Could you check a few things on this model? Use its own coordinates, in mm. Face numbers are marked on the shaded views. A direction names the side the tool comes from. Round coordinates to 2 decimals unless told otherwise and drop trailing zeros. Order: outer loops, then holes, each group sorted by start corner. A loop starts at its lowest first (then second) coordinate and runs counter-clockwise, first axis right, second up.
```python
from build123d import *

# Parameters (mm, degrees)
SKETCH1_R           = 1.5
BOSS_EXTRUDE1_DEPTH = 2.5
BOSS_EXTRUDE2_DEPTH = 13
SKETCH3_R           = 1.6
CUT_EXTRUDE1_DEPTH  = 13


with BuildPart() as part:
    # Sketch1 → Boss-Extrude1 (new body)
    with BuildSketch(Plane(origin=(0, 0, 0), x_dir=(1, 0, 0), z_dir=(0, 1, 0))):
        Polygon((-58.606798355, 6.5), (-34.466582946, 0), (112.252986236, 0), (136.393201645, 6.5), (136.393201645, 13), (-58.606798355, 13), align=None)
        with Locations((-11.606798355, 9.25)):
            Circle(SKETCH1_R, mode=Mode.SUBTRACT)
        with Locations((89.393201645, 9.25)):
            Circle(SKETCH1_R, mode=Mode.SUBTRACT)
    extrude(amount=BOSS_EXTRUDE1_DEPTH)

    # Sketch2 → Boss-Extrude2 (add)
    with BuildSketch(Plane(origin=(0, 2.5, 0), x_dir=(1, 0, 0), z_dir=(0, 1, 0))):
        Polygon((-58.606798355, 6.5), (-34.466582946, 0), (10.033417054, 0), (10.033417054, 2.5), (-34.135896564, 2.5), (-57.956798355, 8.914021541), align=None)
        Polygon((136.393201645, 6.5), (112.252986236, 0), (67.752986236, 0), (67.752986236, 2.5), (111.922299855, 2.5), (135.743201645, 8.914021541), align=None)
    extrude(amount=BOSS_EXTRUDE2_DEPTH)

    # Sketch3 → Cut-Extrude1 (cut)
    with BuildSketch(Plane.XY):
        with Locations((-30.716582946, 9)):
            Circle(SKETCH3_R)
        with Locations((6.283417054, 9)):
            Circle(SKETCH3_R)
        with Locations((71.502986236, 9)):
            Circle(SKETCH3_R)
        with Locations((108.502986236, 9)):
            Circle(SKETCH3_R)
    extrude(amount=-CUT_EXTRUDE1_DEPTH, mode=Mode.SUBTRACT)


solid = part.part
```
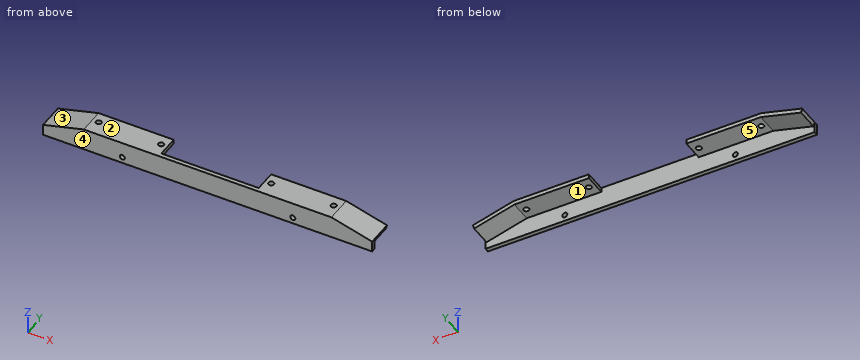
Q1. Imagine slicing it at A-A, the plane y = 9. Please give me the cut outline in (x, z), then the cut area to 3 significant figures.
Q2. I need wall thicknesses on L1, parallel to X at y = 1.3, z = -9.25; L2, parallel to Y at x = 98, z = -8.25; L3, parallel to Z at x = 74.5, y = 4.25. Which ranges of each line are inside material? Lowest first, please.
Q3. For the marked faces 1 and 2, which set-ups out of +Z, -Z, +X, -X, +Y, -Y let a thin tool reach every point of the face, with its end or its side?
Q4. Imagine slicing it at C-C, the plane x = 31.5. Please give me the cut outline in (y, z), then the cut area to 3 significant figures.
Q5. For P1, Ø4, axis at x = 19.5, z = -6, coming from the +Y side; P2, Ø1, axis at x = 106.5, y = 5, coming from the +Z side; P3, Ø6.5, axis at x = 100.5, y = 10, coming from the -Z side, each with a flat end and sliding along its axis, tell me the tip position at first contact or that it passes through.
Q6. Imagine slicing it at D-D, the plane x = -37. Please give me the cut outline in (y, z).
Q7. We'd pull the mould along X, two halves only. Please class the marked faces 3, 4 and 5: released by +X, released by -X, zero draft, split by the parting line, or undercut.
Q8. Imagine slicing it at B-B, the plane x = 95. Please give me the cut outline in (y, z), then the cut area to 3 significant figures.
Filled in:
1. outline: (-58.61, -6.5) - (-57.96, -8.91) - (-34.14, -2.5) - (-32.32, -2.5) - (-32.32, 0) - (-34.47, 0) - close; (-29.12, -2.5) - (4.68, -2.5) - (4.68, 0) - (-29.12, 0) - close; (7.88, -2.5) - (10.03, -2.5) - (10.03, 0) - (7.88, 0) - close; (67.75, -2.5) - (69.9, -2.5) - (69.9, 0) - (67.75, 0) - close; (73.1, -2.5) - (106.9, -2.5) - (106.9, 0) - (73.1, 0) - close; (110.1, -2.5) - (111.92, -2.5) - (135.74, -8.91) - (136.39, -6.5) - (112.25, 0) - (110.1, 0) - close
1. area: 314 mm2
2. L1: x = -58.61 to -13.11, -10.11 to 87.89, 90.89 to 136.39
2. L2: y = 0 to 2.5
2. L3: z = -2.5 to 0
3. face 1: -Z, +Y
3. face 2: +Z, +X, -X, +Y, -Y
4. outline: (0, -13) - (2.5, -13) - (2.5, 0) - (0, 0) - close
4. area: 32.5 mm2
5. P1: stops at y = 2.5
5. P2: stops at z = 0
5. P3: stops at z = -2.5
6. outline: (0, -13) - (2.5, -13) - (2.5, -3.27) - (15.5, -3.27) - (15.5, -0.68) - (0, -0.68) - close
7. face 3: released by -X
7. face 4: zero draft
7. face 5: undercut
8. outline: (0, -13) - (2.5, -13) - (2.5, -2.5) - (15.5, -2.5) - (15.5, 0) - (0, 0) - close
8. area: 65.0 mm2
